Check sheet for the modelled part. Datum: model origin and axes. Units: mm. Face numbers are marked on the shaded views. A direction names the side the tool comes from. Coordinates: 2 decimals unless noted, no trailing zeros. Write each loop counter-clockwise with the first axis right and the second up, starting at its lowest first coordinate (ties: lowest second). Pieces come first, ordered by that corner, then holes. Notation, with made-up numbers: M 60.25,-21 L 117.25,-21 A15 cw 117.25,8 Z; hole C 32.25,39.25 d11. An arc over 180 degrees is marked long. Answer as CSV lines item,"result". Start each with the question number.
Q1. Thickness scan on line 1 along Z through (x, y) = (56, -7.5); line 2 along X through (y, z) = (-1.75, 4); line 3 along Z through (x, y) = (-37, -3.25). Record the ranges inside material, lowest first. Write a range as from..to.
Q2. Sectioned sample at B-B, the plane z = -23. Record the cut outline in (x, y), then the cut area to 3 significant figures.
Q3. Sectioned sample at D-D, the plane y = -8.75. Record the cut outline in (x, z).
Q4. Sectioned sample at A-A, the plane y = -14. Record the cut outline in (x, z).
Q5. Sectioned sample at C-C, the plane x = 21.5. Record the cut outline in (y, z), then the cut area to 3 significant figures.
Q6. Depth check by flat-ended pin: pin 1 Ø8 at (y, z) = (-5, -24.5) entering from -X; pin 2 Ø4 at (y, z) = (-3, -10.5) entering from -X; pin 3 Ø4 at (y, z) = (-5, -14.5) entering from +X. Enter the tip coordinate at first touch or a pass-through.
Q7. Access from +Z, -Z, +X, -X, +Y, -Y to the whole of each face (thin tool, end or side, straight path). Record for the marked faces 1 and 2.
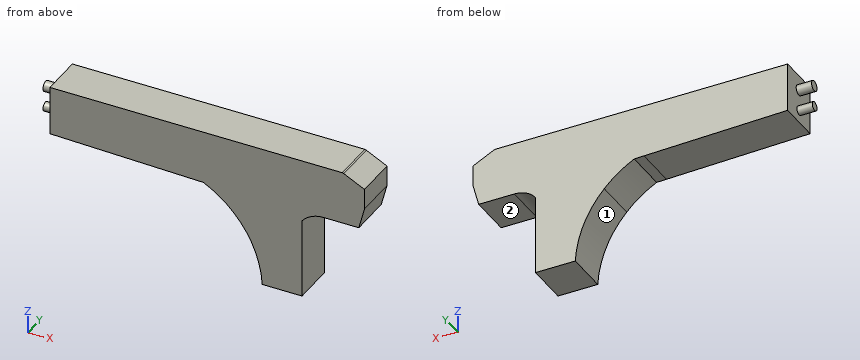
from build123d import *

# Parameters (mm, degrees)
F1_DEPTH = 17.526
F2_R     = 2.11459
F2_R_2   = 1.828308
F3_DEPTH = 6.35


with BuildPart() as f1:
    # F0 (on Front) → F1 (new body)
    with BuildSketch(Plane.XZ):
        with BuildLine():
            ThreePointArc((12.356936, -14.171695), (20.810401, -27.063904), (24.290653, -42.082492))
            Line((24.290653, -42.082492), (40.697493, -42.082492))
            Line((40.697493, -42.082492), (40.697493, -9.268802))
            ThreePointArc((40.697493, -9.268802), (44.57356, -6.129463), (49.433608, -5.007284))
            Line((49.433608, -5.007284), (64.135849, -5.007284))
            Line((64.135849, -5.007284), (66.479683, 3.941904))
            Line((66.479683, 3.941904), (66.479683, 12.464941))
            Line((66.479683, 12.464941), (57.956647, 16.726458))
            Line((57.956647, 16.726458), (57.317417, 16.939534))
            Line((57.317417, 16.939534), (-63.28354, 16.939534))
            Line((-63.28354, 16.939534), (-63.28354, -3.302676))
            Line((-63.28354, -3.302676), (-4.039772, -4.898468))
            Line((-4.039772, -4.898468), (0, -5.007284))
            ThreePointArc((0, -5.007284), (6.582655, -9.044499), (12.356936, -14.171695))
        make_face()
    extrude(amount=F1_DEPTH)

    # F2 (on face) → F3 (join)
    with BuildSketch(Plane(origin=(-63.28354, 0, 0), x_dir=(0, -1, 0), z_dir=(-1, 0, 0))):
        with Locations((8.763, 10.517745)):
            Circle(F2_R)
        with Locations((9.03319, 1.771447)):
            Circle(F2_R_2)
    extrude(amount=F3_DEPTH)


solid = f1.part
Output:
1,line 1,"z = -5.01..16.94"
1,line 2,"x = -63.28..66.48"
1,line 3,"z = -4.01..16.94"
2,outline,"M 18.82,-17.53 L 40.7,-17.53 L 40.7,0 L 18.82,0 Z"
2,area,"383 mm^2"
3,outline,"M -69.63,-0.03 L -63.28,-0.03 L -63.28,-3.3 L -4.04,-4.9 L 0,-5.01 A43.94 cw 12.36,-14.17 A43.94 cw 24.29,-42.08 L 40.7,-42.08 L 40.7,-9.27 A11.09 cw 49.43,-5.01 L 64.14,-5.01 L 66.48,3.94 L 66.48,12.46 L 57.96,16.73 L 57.32,16.94 L -63.28,16.94 L -63.28,12.63 L -69.63,12.63 L -69.63,8.4 L -63.28,8.4 L -63.28,3.58 L -69.63,3.58 Z"
4,outline,"M -63.28,-3.3 L -4.04,-4.9 L 0,-5.01 A43.94 cw 12.36,-14.17 A43.94 cw 24.29,-42.08 L 40.7,-42.08 L 40.7,-9.27 A11.09 cw 49.43,-5.01 L 64.14,-5.01 L 66.48,3.94 L 66.48,12.46 L 57.96,16.73 L 57.32,16.94 L -63.28,16.94 Z"
5,outline,"M -17.53,-28.78 L 0,-28.78 L 0,16.94 L -17.53,16.94 Z"
5,area,"801 mm^2"
6,pin 1,"stops at x = 17.32"
6,pin 2,"stops at x = 5.83"
6,pin 3,"stops at x = 40.7"
7,face 1,"-Z, -X, +Y, -Y"
7,face 2,"-Z, +X, +Y, -Y"
